Solid Edge part; units mm, degrees
sketch "Sketch1" plane through (0, 0, 0) normal (0, 0, 1) x (1, 0, 0)
  line L0 (-120.65, -139.7) -> (120.65, -139.7)
  line L1 (120.65, -139.7) -> (120.65, 139.7)
  line L2 (120.65, 139.7) -> (-120.65, 139.7)
  line L3 (-120.65, 139.7) -> (-120.65, -139.7)
extrude "Protrusion1" add sketch "Sketch1" along normal mid plane 101.6
sketch "Sketch2" plane through (0, -139.7, 0) normal (0, -1, 0) x (1, 0, 0)
  line L0 (-120.65, 50.8) -> (120.65, 50.8)
  line L1 (120.65, 50.8) -> (120.65, 3.175)
  line L2 (120.65, 3.175) -> (-120.65, 3.175)
  line L3 (-120.65, 3.175) -> (-120.65, 50.8)
extrude "Cutout1" cut sketch "Sketch2" against normal up to vertex (279.4 mm away)
shell "Thinwall_1" thickness 38.1 removed faces 1 at (82.8463, 90.3393, 3.175)
fillet "Round_1" radius 12.7 8 edges at (120.65, 139.7, -23.8125) (120.65, -139.7, -23.8125) (-120.65, -139.7, -23.8125) (-120.65, 139.7, -23.8125) (0, -139.7, -50.8) (-120.65, 0, -50.8) (120.65, 0, -50.8) (0, 139.7, -50.8)
fillet "Round_2" radius 6.35 4 edges at (-82.55, 101.6, -4.7625) (82.55, 101.6, -4.7625) (82.55, -101.6, -4.7625) (-82.55, -101.6, -4.7625)
sketch "Sketch3" plane through (0, 0, -50.8) normal (0, 0, -1) x (-1, 0, 0)
  line L0 (54.0978, 0.4438) -> (76.2, 0.4438)
  line L1 (76.2, 0.4438) -> (76.2, -22.3123)
  line L2 (76.2, -22.3123) -> (54.0978, -22.3123)
  line L3 (54.0978, -22.3123) -> (54.0978, 0.4438)
extrude "ExtrudedCutout_6" cut sketch "Sketch3" against normal blind 98.1987
sketch "Sketch4" plane through (0, 0, -50.8) normal (0, 0, -1) x (0, -1, 0)
  line L0 (24.5981, 20.3184) -> (24.5981, -17.6816)
  line L1 (24.5981, -17.6816) -> (-13.4019, -17.6816)
  line L2 (-13.4019, -17.6816) -> (-13.4019, 20.3184)
  line L3 (-13.4019, 20.3184) -> (24.5981, 20.3184)
extrude "ExtrudedCutout_7" cut sketch "Sketch4" against normal blind 83.9753
Verification items for the finished model (mm, model axes). A direction names the side the tool comes from. Round coordinates to 2 decimals unless told otherwise and drop trailing zeros. Write each loop counter-clockwise with the first axis right and the second up, starting at its lowest first coordinate (ties: lowest second). Pieces come first, ordered by that corner, then holes. Notation, with made-up numbers: (30.5, 21) -> (61.5, 21) arc R33 ccw to (61.5, 58) -> close; hole circle Ø1 at (-30, 46.5). An arc over 180 degrees is marked (long way). Write each question's results on one line, items separated by ' | '.
Q1. Thickness scan on probe 1 along Y at (x, z) = (45, -5); probe 2 along X at (y, z) = (-12.5, -14); probe 3 along X at (y, z) = (56, -12). Record the ranges inside material, lowest first.
Derived:
probe 1: y = -139.7 to -101.6, 101.6 to 139.7 | probe 2: x = -120.65 to -76.2, -54.1 to -20.32, 17.68 to 120.65 | probe 3: x = -120.65 to -82.55, 82.55 to 120.65
Q2. Sectioned sample at C-C, the plane z = -9. Record the boundary of the cut face in (x, y).
Derived:
outline: (-120.65, -127) arc R12.7 ccw to (-107.95, -139.7) -> (107.95, -139.7) arc R12.7 ccw to (120.65, -127) -> (120.65, 127) arc R12.7 ccw to (107.95, 139.7) -> (-107.95, 139.7) arc R12.7 ccw to (-120.65, 127) -> close; hole (-82.55, -95.25) arc R6.35 ccw to (-76.2, -101.6) -> (76.2, -101.6) arc R6.35 ccw to (82.55, -95.25) -> (82.55, 95.25) arc R6.35 ccw to (76.2, 101.6) -> (-76.2, 101.6) arc R6.35 ccw to (-82.55, 95.25) -> close
Q3. Go/stop test with flat-tipped pins: pin 1 Ø4 at (x, y) = (-27, 43.5) entering from +Z; pin 2 Ø10 at (x, z) = (-18.5, -38.5) entering from +Y. Record where each tip stops, or that it passes through.
Derived:
pin 1: stops at z = -12.7 | pin 2: stops at y = 139.7
Q4. Sectioned sample at B-B, the plane z = -29. Record the boundary of the cut face in (x, y).
Derived:
outline: (-120.65, -127) arc R12.7 ccw to (-107.95, -139.7) -> (107.95, -139.7) arc R12.7 ccw to (120.65, -127) -> (120.65, 127) arc R12.7 ccw to (107.95, 139.7) -> (-107.95, 139.7) arc R12.7 ccw to (-120.65, 127) -> close; hole (-76.2, -22.31) -> (-54.1, -22.31) -> (-54.1, 0.44) -> (-76.2, 0.44) -> close; hole (-20.32, -24.6) -> (17.68, -24.6) -> (17.68, 13.4) -> (-20.32, 13.4) -> close
Q5. Sectioned sample at A-A, the plane x = 9. Record the boundary of the cut face in (y, z) (3 decimals), and give its area (3 significant figures).
Derived:
outline: (-139.7, -38.1) arc R12.7 ccw to (-127, -50.8) -> (-24.598, -50.8) -> (-24.598, -12.7) -> (-101.6, -12.7) -> (-101.6, 3.175) -> (-139.7, 3.175) -> close; (13.402, -50.8) -> (127, -50.8) arc R12.7 ccw to (139.7, -38.1) -> (139.7, 3.175) -> (101.6, 3.175) -> (101.6, -12.7) -> (13.402, -12.7) -> close | area: 10,300 mm²
Q6. Access from +Z, -Z, +X, -X, +Y, -Y to the whole of each face (thin tool, end or side, straight path). Record for faces 5 (the face through (-20.318, -5, -32)), 6 (the face through (2, 139.7, -18)), 7 (the face through (80.74, 99.69, -4.65)).
Derived:
face 5: +Z, -Z | face 6: +Z, -Z, +X, -X, +Y | face 7: +Z
Q7. Sectioned sample at D-D, the plane y = -63. Record the boundary of the cut face in (x, z) (3 decimals), and give its area (3 significant figures).
Derived:
outline: (-120.65, -38.1) arc R12.7 ccw to (-107.95, -50.8) -> (107.95, -50.8) arc R12.7 ccw to (120.65, -38.1) -> (120.65, 3.175) -> (82.55, 3.175) -> (82.55, -12.7) -> (-82.55, -12.7) -> (-82.55, 3.175) -> (-120.65, 3.175) -> close | area: 10,300 mm²
Q8. Draft check along Y on faces 1 (the face through (17.682, -6, -32)), 2 (the face through (117.03, 1.78, -46.98)), 3 (the face through (-2, -24.598, -32)), 4 (the face through (116.83, -136.08, -17.17)). Enter one of: released by +Y, released by -Y, zero draft, split by the parting line, or undercut.
Derived:
face 1: undercut | face 2: zero draft | face 3: undercut | face 4: released by -Y
